from build123d import *

# Parameters (mm, degrees)
SKETCH1_W           = 438.15
SKETCH1_H           = 381
SKETCH1_W_2         = 381
SKETCH1_H_2         = 323.85
BOSS_EXTRUDE1_DEPTH = 28.575
SKETCH2_R           = 4.7625
CUT_EXTRUDE1_DEPTH  = 582.337211199
SKETCH3_R           = 4.7625
CUT_EXTRUDE2_DEPTH  = 28.575


with BuildPart() as part:
    # Sketch1 → Boss-Extrude1 (new body)
    with BuildSketch(Plane(origin=(0, 0, 0), x_dir=(1, 0, 0), z_dir=(0, 1, 0))):
        with Locations((219.075, -190.5)):
            Rectangle(SKETCH1_W, SKETCH1_H)
        with Locations((219.075, -190.5)):
            Rectangle(SKETCH1_W_2, SKETCH1_H_2, mode=Mode.SUBTRACT)
    extrude(amount=BOSS_EXTRUDE1_DEPTH)

    # Sketch2 → Cut-Extrude1 (cut, through all)
    with BuildSketch(Plane(origin=(0, 0, 0), x_dir=(-1, 0, 0), z_dir=(0, 0, -1))):
        with Locations((-44.45, 14.2875)):
            Circle(SKETCH2_R)
        with Locations((-95.25, 14.2875)):
            Circle(SKETCH2_R)
    extrude(amount=-CUT_EXTRUDE1_DEPTH, mode=Mode.SUBTRACT)

    # Sketch3 → Cut-Extrude2 (cut)
    with BuildSketch(Plane(origin=(0, 28.575, 0), x_dir=(1, 0, 0), z_dir=(0, 1, 0))):
        with Locations(Location((336.55, -14.2875, 0), (0, 0, 270))):
            Circle(SKETCH3_R)
        with Locations(Location((336.55, -366.7125, 0), (0, 0, 90))):
            Circle(SKETCH3_R)
    extrude(amount=-CUT_EXTRUDE2_DEPTH, mode=Mode.SUBTRACT)


solid = part.part
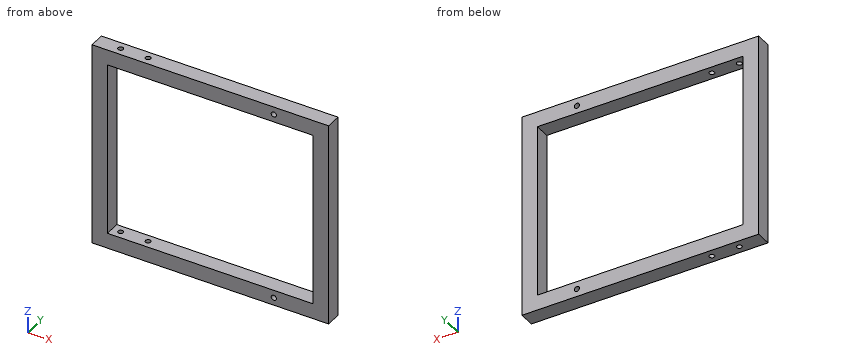
Source: CAD feature listing. Evaluate the final solid. Frame: model axes, mm. Round coordinates to 2 decimals unless told otherwise and drop trailing zeros. Order: outer loops, then holes, each group sorted by start corner. A loop starts at its lowest first (then second) coordinate and runs counter-clockwise, first axis right, second up. Notation, with made-up numbers: (-13.75, -7) - (32.25, -7) arc R30 ccw to (32.25, 24) - close; hole circle Ø6 at (-8.5, 83.5). An arc over 180 degrees is marked (long way). Use a Markdown table: item, result. Add a question column.
1. Line query: probe 1 along Z at (x, y) = (190, 3.5) (3 decimals); probe 2 along X at (y, z) = (2, 108) (3 decimals); probe 3 along Z at (x, y) = (336.55, 11.5) (3 decimals). Output: solid intervals per line, ascending.
2. Section query B-B (x = 355). Return the cut outline in (y, z) (3 decimals).
3. Section query A-A (z = 153). Return the cut outline in (x, y) (3 decimals), then the cut area to 3 significant figures.
Derived:
| question | item | result |
|---|---|---|
| 1 | probe 1 | 0 to 28.575, 352.425 to 381 |
| 1 | probe 2 | 0 to 28.575, 409.575 to 438.15 |
| 1 | probe 3 | 0 to 9.525, 19.05 to 28.575, 352.425 to 361.95, 371.475 to 381 |
| 2 | outline | (0, 0) - (28.575, 0) - (28.575, 28.575) - (0, 28.575) - close; (0, 352.425) - (28.575, 352.425) - (28.575, 381) - (0, 381) - close |
| 3 | outline | (0, 0) - (28.575, 0) - (28.575, 28.575) - (0, 28.575) - close; (409.575, 0) - (438.15, 0) - (438.15, 28.575) - (409.575, 28.575) - close |
| 3 | area | 1,630 mm2 |
